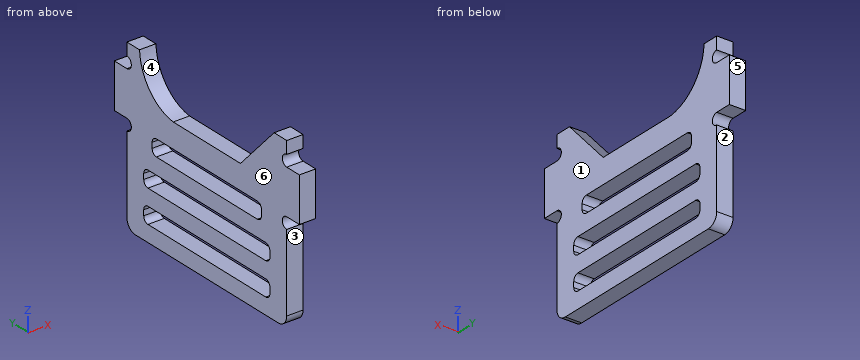
```python
from build123d import *

# Parameters (mm, degrees)
EXTRUDE_1_DEPTH     = 3
SKETCH_4_W          = 14
SKETCH_4_H          = 38
SKETCH_4_W_2        = 3
SKETCH_4_H_2        = 30
EXTRUDE_2_DEPTH     = 3
FILLET_1_R          = 2
SKETCH_5_W          = 3
SKETCH_5_H          = 26
CUT_EXTRUDE_1_DEPTH = 10
FILLET_2_R          = 1


with BuildPart() as part:
    # 草图1 → 凸台-拉伸1 (new body)
    with BuildSketch(Plane(origin=(0, 0, 0), x_dir=(0, 0, -1), z_dir=(1, 0, 0))):
        with BuildLine():
            Line((-4.1, 22), (-4.1, 19))
            ThreePointArc((-4.1, 19), (-5.15, 17.95), (-6.2, 19))
            Line((-6.2, 19), (-8.5, 19))
            Line((-8.5, 19), (-8.5, -19))
            Line((-8.5, -19), (-6.2, -19))
            ThreePointArc((-6.2, -19), (-5.15, -17.95), (-4.1, -19))
            Line((-4.1, -19), (-4.1, -22))
            Line((-4.1, -22), (4.1, -22))
            Line((4.1, -22), (4.1, -19))
            ThreePointArc((4.1, -19), (5.15, -17.95), (6.2, -19))
            Line((6.2, -19), (8.5, -19))
            Line((8.5, -19), (8.5, 19))
            Line((8.5, 19), (6.2, 19))
            ThreePointArc((6.2, 19), (5.15, 17.95), (4.1, 19))
            Line((4.1, 19), (4.1, 22))
            Line((4.1, 22), (-4.1, 22))
        make_face()
    extrude(amount=EXTRUDE_1_DEPTH)

    # 草图4 → 凸台-拉伸2 (add)
    with BuildSketch(Plane(origin=(3, 0, 0), x_dir=(0, 0, -1), z_dir=(1, 0, 0))):
        with Locations((15.5, 0)):
            Rectangle(SKETCH_4_W, SKETCH_4_H)
        with Locations((12, 0)):
            Rectangle(SKETCH_4_W_2, SKETCH_4_H_2, mode=Mode.SUBTRACT)
        with Locations((18, 0)):
            Rectangle(SKETCH_4_W_2, SKETCH_4_H_2, mode=Mode.SUBTRACT)
    extrude(amount=-EXTRUDE_2_DEPTH)

    # 圆角1
    fillet_1_edges = [part.edges().sort_by_distance(p)[0] for p in [
        (1.5, -19, -22.5),
        (1.5, 19, -22.5),
    ]]
    fillet(fillet_1_edges, radius=FILLET_1_R)

    # 草图5 → 切除-拉伸1 (cut)
    with BuildSketch(Plane(origin=(3, 0, 0), x_dir=(0, 0, -1), z_dir=(1, 0, 0))):
        with BuildLine():
            Line((-8.5, -16), (0, -8))
            Line((0, -8), (0, 8))
            ThreePointArc((0, 8), (-2.777216236, 13.564832749), (-8.5, 16))
            Line((-8.5, 16), (-8.5, -16))
        make_face()
        with Locations((6, 0)):
            Rectangle(SKETCH_5_W, SKETCH_5_H)
    extrude(amount=-CUT_EXTRUDE_1_DEPTH, mode=Mode.SUBTRACT)

    # 圆角2
    fillet_2_edges = [part.edges().sort_by_distance(p)[0] for p in [
        (1.5, 13, -4.5),
        (1.5, 13, -7.5),
        (1.5, -13, -7.5),
        (1.5, -13, -4.5),
        (1.5, -15, -16.5),
        (1.5, -15, -19.5),
        (1.5, 15, -19.5),
        (1.5, 15, -16.5),
        (1.5, -15, -10.5),
        (1.5, -15, -13.5),
        (1.5, 15, -13.5),
        (1.5, 15, -10.5),
    ]]
    fillet(fillet_2_edges, radius=FILLET_2_R)


solid = part.part
```
Can you work these out from the model? Positions are in its coordinate system, mm. Face numbers are marked on the shaded views. A direction names the side the tool comes from. Give positions to 0.01 mm unless a question says otherwise; leave off trailing zeros. Write each loop counter-clockwise with the first axis right and the second up, starting at its lowest first coordinate (ties: lowest second). Pieces come first, ordered by that corner, then holes. Notation, with made-up numbers: (10.5, 38) - (47.5, 38) arc R5 cw to (47.5, 47) - close; hole circle Ø5 at (-17, 34). An arc over 180 degrees is marked (long way). Write item = value, one per line. Start each with the question number.
1. For pin 1 (1 mm diameter, centred on x = 1.5, y = -9, fed in from +Z); pin 2 (0.9 mm diameter, centred on x = 1.5, y = -21, fed in from +Z); pin 3 (1.5 mm diameter, centred on x = 2, z = -12.5, fed in from +Y), each with a flat end and sliding along its axis, tell me the tip position at first contact or that it passes through.
2. Imagine slicing it at A-A (y = -10). Please give me the cut outline in (x, z) (3 decimals), and give its area (3 significant figures).
3. On a 3-axis mill with a long thin cutter (end or side, diameter ignored), from which of +Z, -Z, +X, -X, +Y, -Y can I reach the whole of each face in a straight line? I mean the marked faces 1 and 2. Say none if no direction works.
4. Thinking about a two-plate mould opening in Y: for the marked faces 3, 4, 5 and 6, which applies, released by +Y, released by -Y, zero draft, split by the parting line, or undercut?
5. Imagine slicing it at B-B (z = 5). Please give me the cut outline in (x, y), and give its area (3 significant figures).
6. Imagine slicing it at D-D (z = -14). Please give me the cut outline in (x, y), and give its area (3 significant figures).
7. Please list where these lines run through material, in increasing order: line 1 (Z direction, x = 0.85, y = 3); line 2 (Y direction, x = 1.65, z = -18); line 3 (Z direction, x = 0.25, y = -8.5).
8. Imagine slicing it at C-C (x = 1.4). Count the separate pieces of the cut face and the enclosed holes in it, and give its area (3 significant figures).
Worked answers:
q1.pin_1 = 1.59
q1.pin_2 = 4.1
q1.pin_3 = 19
q2.outline = (0, -22.5) - (3, -22.5) - (3, -19.5) - (0, -19.5) - close; (0, -16.5) - (3, -16.5) - (3, -13.5) - (0, -13.5) - close; (0, -10.5) - (3, -10.5) - (3, -7.5) - (0, -7.5) - close; (0, -4.5) - (3, -4.5) - (3, 2.125) - (0, 2.125) - close
q2.area = 46.9 mm2
q3.face_1 = +Z, -Z, +X, +Y, -Y
q3.face_2 = -Z, +X, -X, +Y
q4.face_3 = released by -Y
q4.face_4 = undercut
q4.face_5 = released by +Y
q4.face_6 = zero draft
q5.outline = (0, -17.96) - (3, -17.96) - (3, -12.71) - (0, -12.71) - close; (0, 15.1) - (3, 15.1) - (3, 17.96) - (0, 17.96) - close
q5.area = 24.3 mm2
q6.outline = (0, -19) - (3, -19) - (3, 19) - (0, 19) - close
q6.area = 114 mm2
q7.line_1 = -22.5 to -19.5, -16.5 to -13.5, -10.5 to -7.5, -4.5 to 0
q7.line_2 = -19 to -15, 15 to 19
q7.line_3 = -22.5 to -19.5, -16.5 to -13.5, -10.5 to -7.5, -4.5 to 0.53
q8.separate_pieces = 1
q8.enclosed_holes = 3
q8.area = 742 mm2
